Verification items for the finished model (mm, model axes). Face numbers are marked on the shaded views. Give positions to 0.01 mm unless a question says otherwise; leave off trailing zeros. Order: outer loops, then holes, each group sorted by start corner. A loop starts at its lowest first (then second) coordinate and runs counter-clockwise, first axis right, second up. Notation, with made-up numbers: (50, 25.5) - (57, 25.5) arc R16 cw to (57, 53.5) - close; hole circle Ø8 at (88, -37.75). An arc over 180 degrees is marked (long way). Answer as a JSON object with one key per item and string values. Group by question number.
(1) Depth check by flat-ended pin: pin 1 Ø0.9 at (x, z) = (73, 0) entering from -Y; pin 2 Ø0.9 at (y, z) = (-31, 0.5) entering from +X; pin 3 Ø1.5 at (x, z) = (33, 0) entering from -Y. Enter the tip coordinate at first touch or a pass-through.
(2) Thickness scan on line 1 (Y direction, x = -28, z = 1.25); line 2 (X direction, y = 26, z = -0.1). Record the ranges inside material, lowest first.
(3) Mould release check, pull along Z, two halves, no side actions. Record for the marked faces 1 and 2: +Z half, -Z half, draft (parallel to the pull), parting line (faces both ways), or undercut.
(4) Section check B-B (x = 28). Record the boundary of the cut face in (y, z).
(5) Section check A-A (z = 0.4). Record the boundary of the cut face in (x, y).
(6) Section check C-C (y = -34.5). Record the boundary of the cut face in (x, z).
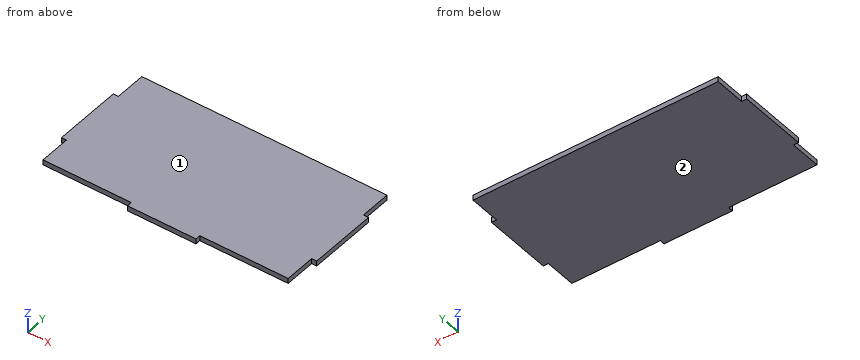
```python
from build123d import *

# Parameters (mm, degrees)
SKETCH1_W           = 143.2306
SKETCH1_H           = 76.2
BOSS_EXTRUDE1_DEPTH = 1.4986
SKETCH2_W           = 2.9464
SKETCH2_H           = 40
SKETCH2_W_2         = 40
SKETCH2_H_2         = 2.9464
BOSS_EXTRUDE2_DEPTH = 2.9972


with BuildPart() as part:
    # Sketch1 → Boss-Extrude1 (new body, symmetric)
    with BuildSketch(Plane.XY):
        Rectangle(SKETCH1_W, SKETCH1_H)
    extrude(amount=BOSS_EXTRUDE1_DEPTH, both=True)

    # Sketch2 → Boss-Extrude2 (add, through all)
    with BuildSketch(Plane.XY.offset(1.4986)):
        with Locations((-73.0885, 0)):
            Rectangle(SKETCH2_W, SKETCH2_H)
        with Locations((0, -39.5732)):
            Rectangle(SKETCH2_W_2, SKETCH2_H_2)
        with Locations((73.0885, 0)):
            Rectangle(SKETCH2_W, SKETCH2_H)
    extrude(amount=-BOSS_EXTRUDE2_DEPTH)


solid = part.part
```
Solutions:
{
 "1": {"pin 1": "stops at y = -20", "pin 2": "stops at x = 71.62", "pin 3": "stops at y = -38.1"},
 "2": {"line 1": "y = -38.1 to 38.1", "line 2": "x = -71.62 to 71.62"},
 "3": {"face 1": "+Z half", "face 2": "-Z half"},
 "4": {"outline": "(-38.1, -1.5) - (38.1, -1.5) - (38.1, 1.5) - (-38.1, 1.5) - close"},
 "5": {"outline": "(-74.56, -20) - (-71.62, -20) - (-71.62, -38.1) - (-20, -38.1) - (-20, -41.05) - (20, -41.05) - (20, -38.1) - (71.62, -38.1) - (71.62, -20) - (74.56, -20) - (74.56, 20) - (71.62, 20) - (71.62, 38.1) - (-71.62, 38.1) - (-71.62, 20) - (-74.56, 20) - close"},
 "6": {"outline": "(-71.62, -1.5) - (71.62, -1.5) - (71.62, 1.5) - (-71.62, 1.5) - close"}
}
